The model under review builds one solid part; all positions refer to its coordinate system, in mm. A direction names the side the tool comes from. Coordinates: 2 decimals unless noted, no trailing zeros. Loops run counter-clockwise (first coordinate to the right, second up) from the corner with the lowest first, then second, coordinate; pieces in that order, holes last. Notation, with made-up numbers: M 13.25,28.5 L 34.25,28.5 A11 cw 34.25,48.5 Z; hole C 55.5,69 d3. An arc over 180 degrees is marked long. Write item = value, one per line. Start each with the question number.
Q1. Mouldability with a two-part tool opening along X and no side actions: class faces 1 (the face through (-7, 49, 1)), 2 (the face through (7, 1, 1)), 3 (the face through (7, 7, 1)), 4 (the face through (0, 25, 3)) as released by +X, released by -X, zero draft, split by the parting line, or undercut.
Q2. We need section A-A on x = 2.5. Give the boundary of the cut face in (y, z).
Q3. We need section C-C on x = -5.75. Give the boundary of the cut face in (y, z), and give its area (3 significant figures).
Q4. We need section B-B on z = 0.8. Count the separate pieces of the cut face and the enclosed holes in it, and give its area (3 significant figures).
Q5. Wall thickness on probe 1 along Y at (x, z) = (-3.5, 2.5); probe 2 along X at (y, z) = (6, 1.4); probe 3 along Y at (x, z) = (-6.5, 0.85): over which ranges is each line inside the solid? List them lowest first.
Q6. For faces 5 (the face through (0, 17.2, 1)), 6 (the face through (0, 0, 1)), list the 3-axis set-ups (+Z, -Z, +X, -X, +Y, -Y) from which the entire face can be reached by the end or side of a thin tool; tool diameter is ignored.
from build123d import *

# Parameters (mm, degrees)
F1_DEPTH = 3


with BuildPart() as f1:
    # F0 (on Top) → F1 (new body)
    with BuildSketch(Plane.XY):
        with BuildLine():
            Line((4, 50), (-4, 50))
            ThreePointArc((-4, 50), (-7.535534, 48.535534), (-9, 45))
            Line((-9, 45), (-9, 5))
            ThreePointArc((-9, 5), (-7.535534, 1.464466), (-4, 0))
            Line((-4, 0), (4, 0))
            ThreePointArc((4, 0), (7.535534, 1.464466), (9, 5))
            Line((9, 5), (9, 45))
            ThreePointArc((9, 45), (7.535534, 48.535534), (4, 50))
        make_face()
        with BuildLine():
            ThreePointArc((-7, 7.95), (-7.176777, 8.376777), (-6.75, 8.2))
            Line((-6.75, 8.2), (6.75, 8.2))
            ThreePointArc((6.75, 8.2), (7, 8.45), (7.25, 8.2))
            ThreePointArc((7.25, 8.2), (7.176777, 8.023223), (7, 7.95))
            Line((7, 7.95), (7, 5.25))
            ThreePointArc((7, 5.25), (7.176777, 5.176777), (7.25, 5))
            ThreePointArc((7.25, 5), (7, 4.75), (6.75, 5))
            Line((6.75, 5), (-6.75, 5))
            ThreePointArc((-6.75, 5), (-7.176777, 4.823223), (-7, 5.25))
            Line((-7, 5.25), (-7, 7.95))
        make_face(mode=Mode.SUBTRACT)
        with BuildLine():
            ThreePointArc((-7, 16.95), (-7.176777, 17.376777), (-6.75, 17.2))
            Line((-6.75, 17.2), (6.75, 17.2))
            ThreePointArc((6.75, 17.2), (7, 17.45), (7.25, 17.2))
            ThreePointArc((7.25, 17.2), (7.176777, 17.023223), (7, 16.95))
            Line((7, 16.95), (7, 14.25))
            ThreePointArc((7, 14.25), (7.176777, 14.176777), (7.25, 14))
            ThreePointArc((7.25, 14), (7, 13.75), (6.75, 14))
            Line((6.75, 14), (-6.75, 14))
            ThreePointArc((-6.75, 14), (-7.176777, 13.823223), (-7, 14.25))
            Line((-7, 14.25), (-7, 16.95))
        make_face(mode=Mode.SUBTRACT)
        with BuildLine():
            ThreePointArc((-7, 44.75), (-7.176777, 45.176777), (-6.75, 45))
            Line((-6.75, 45), (6.75, 45))
            ThreePointArc((6.75, 45), (7, 45.25), (7.25, 45))
            ThreePointArc((7.25, 45), (7.176777, 44.823223), (7, 44.75))
            Line((7, 44.75), (7, 42.05))
            ThreePointArc((7, 42.05), (7.176777, 41.976777), (7.25, 41.8))
            ThreePointArc((7.25, 41.8), (7, 41.55), (6.75, 41.8))
            Line((6.75, 41.8), (-6.75, 41.8))
            ThreePointArc((-6.75, 41.8), (-7.176777, 41.623223), (-7, 42.05))
            Line((-7, 42.05), (-7, 44.75))
        make_face(mode=Mode.SUBTRACT)
    extrude(amount=F1_DEPTH)


solid = f1.part
Returned:
q1.face_1 = released by -X
q1.face_2 = released by +X
q1.face_3 = undercut
q1.face_4 = zero draft
q2.outline = M 0,0 L 5,0 L 5,3 L 0,3 Z; M 8.2,0 L 14,0 L 14,3 L 8.2,3 Z; M 17.2,0 L 41.8,0 L 41.8,3 L 17.2,3 Z; M 45,0 L 50,0 L 50,3 L 45,3 Z
q3.outline = M 0.32,0 L 5,0 L 5,3 L 0.32,3 Z; M 8.2,0 L 14,0 L 14,3 L 8.2,3 Z; M 17.2,0 L 41.8,0 L 41.8,3 L 17.2,3 Z; M 45,0 L 49.68,0 L 49.68,3 L 45,3 Z
q3.area = 119 mm^2
q4.separate_pieces = 1
q4.enclosed_holes = 3
q4.area = 742 mm^2
q5.probe_1 = 0 to 5, 8.2 to 14, 17.2 to 41.8, 45 to 50
q5.probe_2 = -9 to -7, 7 to 9
q5.probe_3 = 0.67 to 5, 8.2 to 14, 17.2 to 41.8, 45 to 49.33
q6.face_5 = +Z, -Z
q6.face_6 = +Z, -Z, +X, -X, -Y
